Check sheet for the modelled part. Datum: model origin and axes. Units: mm. A direction names the side the tool comes from. Round coordinates to 2 decimals unless told otherwise and drop trailing zeros. Write each loop counter-clockwise with the first axis right and the second up, starting at its lowest first coordinate (ties: lowest second). Pieces come first, ordered by that corner, then holes.
Item 1: Depth check by flat-ended pin: pin 1 (2 mm diameter, centred on y = 0.5, z = -4.5, fed in from +X); pin 2 (2.5 mm diameter, centred on x = 0, z = -4.5, fed in from +Y). Enter the tip coordinate at first touch or a pass-through.
Item 2: Material ranges on line 1 along Z through (x, y) = (0, -1.8); line 2 along Z through (x, y) = (-0.5, 1.75); line 3 along X through (y, z) = (2.05, -51.3), recorded low to high.
Item 3: Section check A-A, the plane z = -51.3. Record the cut outline in (x, y), plus the area to 3 significant figures.
Item 4: Section check C-C, the plane z = -35.5. Record the cut outline in (x, y), plus the area to 3 significant figures.
Item 5: Section check D-D, the plane y = -0.5. Record the cut outline in (x, z), plus the area to 3 significant figures.
Item 6: Section check B-B, the plane x = 1. Record the cut outline in (y, z).
Item 7: Release check for a two-part mould opening along Z. For faces 1 (the flat face through (-1, 1.25, -3)), 2 (the flat face through (0, -2, -55.8)), 3 (the cylindrical face through (-0.325, -2.655, -49.836)) record: pulls with the +Z half, pulls with the -Z half, needs draft (parallel to the pull), parting line crosses it, or undercut.
Item 8: Set-up check for faces 4 (the flat face through (2.8, 0, -3)), 5 (the flat face through (3.534, 2.079, -27.509)), 6 (the flat face through (-1, 1.25, -53)): record each of +Z, -Z, +X, -X, +Y, -Y from which the full face is reachable in a straight line by a thin tool's end or side.
Autodesk Inventor part; units mm, degrees
ref_plane "Work Plane1" through (0, 0, -27.9) normal (0, 0, -1) x (-1, 0, 0)
ref_plane "YZ Plane" through (0, 0, 0) normal (1, 0, 0) x (0, 1, 0)
ref_plane "XZ Plane" through (0, 0, 0) normal (0, 1, 0) x (-1, 0, 0)
sketch "Sketch1" plane through (0, 0, 0) normal (0, 0, 1) x (1, 0, 0)
  line L0 (-2.3671, -4.1) -> (-4.7343, 0)
  line L1 (-4.7343, 0) -> (-2.3671, 4.1)
  line L2 (-2.3671, 4.1) -> (2.3671, 4.1)
  line L3 (2.3671, 4.1) -> (4.7343, 0)
  line L4 (4.7343, 0) -> (2.3671, -4.1)
  line L5 (2.3671, -4.1) -> (-2.3671, -4.1)
  point P0 (0, 0)
  point P1 (0, 0)
  dimension "d0" = 4.1
extrude "Extrusion1" add sketch "Sketch1" against normal blind 55.8
sketch "Sketch2" plane through (4.7343, 0, 0) normal (0.866, 0.5, 0) x (0, 0, -1)
  line L0 (0, 4.7343) -> (0, 0)
  line L1 (4.75, 5.1671) -> (7.25, 5.1671)
  line L2 (7.25, 5.1671) -> (7.25, -0.4329)
  line L3 (7.25, -0.4329) -> (4.75, -0.4329)
  line L4 (4.75, -0.4329) -> (4.75, 5.1671)
  line L5 (4.75, 5.1671) -> (7.25, -0.4329) construction
  line L6 (7.25, 5.1671) -> (4.75, -0.4329) construction
  point P0 (0, 2.3671)
  point P1 (6, 2.3671)
  dimension "d3" = 2.5
  dimension "d4" = 5.6
  dimension "d10" = 0
  dimension "d11" = 6
extrude "Extrusion2" [suppressed]
sketch "Sketch3" plane through (0, 0, 0) normal (0, 0, 1) x (1, 0, 0)
  circle A0 centre (0, 0) radius 1.5
  dimension "d7" = 3
extrude "Extrusion3" [suppressed]
ref_plane "Work Plane1" through (0, 0, -27.9) normal (0, 0, -1) x (-1, 0, 0)
mirror "Mirror1" [suppressed]
sketch "Sketch4" plane through (1.5014, 4.1, -7.25) normal (0, 0, 1) x (1, 0, 0)
  line L0 (0, 0) -> (-4.5469, -2.6251)
  line L1 (-1.7469, -7.4749) -> (-4.5469, -2.6251)
  line L2 (2.8, -4.8497) -> (-1.7469, -7.4749)
  line L3 (-4.5469, -2.6251) -> (-4.5469, -5.8583)
  line L4 (-1.7469, -7.4749) -> (-4.5469, -5.8583)
  line L5 (-1.7469, -7.4749) -> (-4.5469, -2.6251)
  point P0 (-1.5014, -4.1)
  dimension "d12" = 120
  dimension "d13" = 120
extrude "Extrusion4" [suppressed]
sketch "Sketch5" plane through (-4.7343, 0, -55.8) normal (-0.866, -0.5, 0) x (0, 0, 1)
  line L0 (0, -4.7343) -> (0, 0)
  line L1 (4.75, 0.4331) -> (7.25, 0.4331)
  line L2 (7.25, 0.4331) -> (7.25, -5.1669)
  line L3 (7.25, -5.1669) -> (4.75, -5.1669)
  line L4 (4.75, -5.1669) -> (4.75, 0.4331)
  line L5 (4.75, 0.4331) -> (7.25, -5.1669) construction
  line L6 (7.25, 0.4331) -> (4.75, -5.1669) construction
  line L7 (0, -3.8671) -> (0, -0.8671)
  line L8 (0, -4.7343) -> (0, 0)
  line L9 (0, 0) -> (0, 2.3671)
  line L10 (0, 2.3671) -> (0, 0)
  line L11 (0, 0) -> (0, -4.7343)
  line L12 (0, -4.7343) -> (0, -7.1014)
  line L13 (0, -7.1014) -> (0, -4.7343)
  line L14 (9.5, -0.8671) -> (9.5, -3.8671)
  line L15 (0, -3.8671) -> (0, -0.8671)
  line L16 (55.8, -7.1014) -> (0, -7.1014)
  line L17 (55.8, 2.3671) -> (0, 2.3671)
  point P0 (55.8, -2.3671)
  point P1 (6, -2.3669)
  dimension "d16" = 2.5
  dimension "d17" = 5.6
  dimension "d18" = 6
  dimension "d25" = 1.9345
extrude "Extrusion5" [suppressed]
sketch "Sketch6" plane through (-1.5019, -4.1, -42.75) normal (0, 0, -1) x (-1, 0, 0)
  line L0 (-1.7472, 7.4751) -> (-4.5472, 2.6253)
  line L1 (-4.5472, 2.6253) -> (-4.5472, 5.8585)
  line L2 (-1.7472, 7.4751) -> (-4.5472, 5.8585)
  line L3 (2.7993, 4.8501) -> (-1.7472, 7.4751)
  line L4 (0, 0) -> (-4.5472, 2.6253)
  line L5 (-1.7472, 7.4751) -> (-4.5472, 2.6253)
  point P0 (-1.5019, 4.1)
  dimension "d21" = 120
  dimension "d22" = 120
extrude "Extrusion6" [suppressed]
sketch "Sketch8" plane through (0, 0, -55.8) normal (0, 0, -1) x (-1, 0, 0)
  line L0 (-2.8, 1.25) -> (2.8, 1.25)
  line L1 (2.8, 1.25) -> (2.8, -1.25)
  line L2 (2.8, -1.25) -> (-2.8, -1.25)
  line L3 (-2.8, -1.25) -> (-2.8, 1.25)
  line L4 (-2.8, 1.25) -> (2.8, -1.25) construction
  line L5 (2.8, 1.25) -> (-2.8, -1.25) construction
  point P0 (0, 0)
  dimension "d32" = 5.6
  dimension "d33" = 2.5
  dimension "d46" = 1.25
  dimension "d47" = 2.8
extrude "Extrusion8" cut sketch "Sketch8" against normal blind 6.5
sketch "Sketch9" plane through (-2.3671, 4.1, 0) normal (0, 1, 0) x (1, 0, 0)
  line L0 (4.7343, 0) -> (4.7343, 55.8)
  line L1 (0, 55.8) -> (4.7343, 55.8)
  line L2 (0, 0) -> (0, 55.8)
  line L3 (0, 0) -> (4.7343, 0)
  line L4 (5.1671, 55.8) -> (-0.4329, 55.8)
  line L5 (2.3671, 55.8) -> (2.3671, 0) construction
  line L6 (2.3671, 55.8) -> (58.1671, 55.8) construction
  circle A0 centre (2.3671, 51.3) radius 1.5
  dimension "d36" = 90
  dimension "d37" = 3
  dimension "d38" = 0
  dimension "d39" = 4.5
extrude "Extrusion9" cut sketch "Sketch9" against normal up to surface (8.2 mm away) contours A0
sketch "Sketch10" plane through (-2.8, 1.25, -55.8) normal (0, -1, 0) x (1, 0, 0)
  circle A0 centre (2.8, 4.5) radius 1.5
  line L0 (5.6, 0) -> (0, 0)
  line L1 (5.6, 0) -> (5.6, 6.5)
  line L2 (5.6, 6.5) -> (0, 6.5)
  line L3 (0, 0) -> (0, 6.5)
  line L4 (0, 6.5) -> (2.8, 8.1166)
  line L5 (0, 6.5) -> (3.9156, 6.5) construction
  line L6 (5.6, 6.5) -> (2.8, 8.1166)
  line L7 (5.6, 6.5) -> (8.8332, 6.5) construction
  line L8 (5.6, 6.5) -> (0, 6.5)
  point P0 (2.8, 55.8)
  dimension "d42" = 30
  dimension "d43" = 150
extrude "Extrusion10" cut sketch "Sketch10" along normal blind 2.5 contours L2 L4 L6
mirror "Mirror3" about plane through (0, 0, -27.9) normal (0, 0, -1) of "Extrusion8", "Extrusion9", "Extrusion10"
properties part number "SupportFirstToSecond" material "ABS Plastic"
Values found:
1. pin 1: stops at x = 4.73
1. pin 2: passes through
2. line 1: z = -55.8 to -52.8, -49.8 to -6, -3 to 0
2. line 2: z = -55.8 to -52.71, -49.89 to -5.91, -3.09 to 0
2. line 3: x = -3.55 to -1.5, 1.5 to 3.55
3. outline: (-4.73, 0) - (-2.37, -4.1) - (-1.5, -4.1) - (-1.5, -1.25) - (-2.8, -1.25) - (-2.8, 1.25) - (-1.5, 1.25) - (-1.5, 4.1) - (-2.37, 4.1) - close; (1.5, -4.1) - (2.37, -4.1) - (4.73, 0) - (2.37, 4.1) - (1.5, 4.1) - (1.5, 1.25) - (2.8, 1.25) - (2.8, -1.25) - (1.5, -1.25) - close
3. area: 27.1 mm2
4. outline: (-4.73, 0) - (-2.37, -4.1) - (2.37, -4.1) - (4.73, 0) - (2.37, 4.1) - (-2.37, 4.1) - close
4. area: 58.2 mm2
5. outline: (-4.45, -55.8) - (-2.8, -55.8) - (-2.8, -49.3) - (0, -47.68) - (2.8, -49.3) - (2.8, -55.8) - (4.45, -55.8) - (4.45, 0) - (2.8, 0) - (2.8, -6.5) - (0, -8.12) - (-2.8, -6.5) - (-2.8, 0) - (-4.45, 0) - close
5. area: 414 mm2
6. outline: (-4.1, -55.8) - (-1.25, -55.8) - (-1.25, -52.42) - (-4.1, -52.42) - close; (-4.1, -50.18) - (-1.25, -50.18) - (-1.25, -48.26) - (1.25, -48.26) - (1.25, -50.18) - (4.1, -50.18) - (4.1, -5.62) - (1.25, -5.62) - (1.25, -7.54) - (-1.25, -7.54) - (-1.25, -5.62) - (-4.1, -5.62) - close; (-4.1, -3.38) - (-1.25, -3.38) - (-1.25, 0) - (-4.1, 0) - close; (1.25, -55.8) - (4.1, -55.8) - (4.1, -52.42) - (1.25, -52.42) - close; (1.25, -3.38) - (4.1, -3.38) - (4.1, 0) - (1.25, 0) - close
7. face 1: needs draft
7. face 2: pulls with the -Z half
7. face 3: undercut
8. face 4: +Z
8. face 5: +Z, -Z, +X, +Y
8. face 6: -Z
